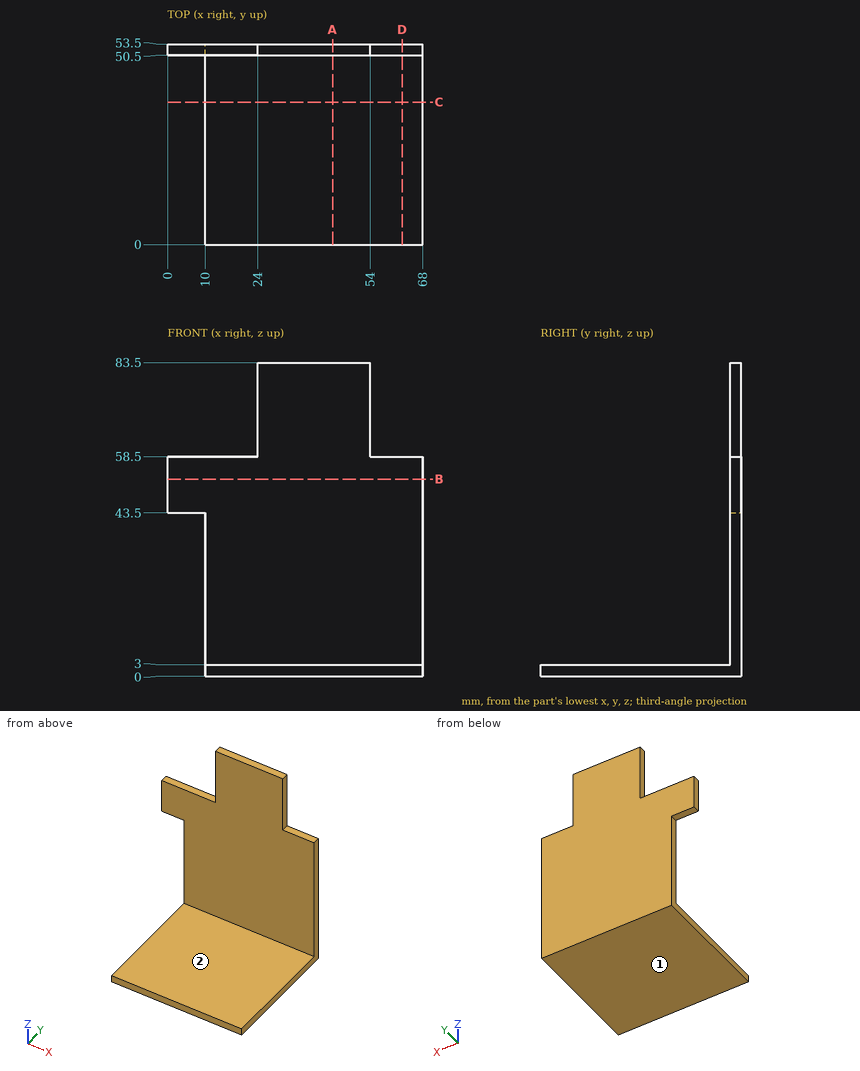
Check sheet for the drawn part. Datum: minimum x, y, z corner. Units: mm. A direction names the side the tool comes from. Give positions to 0.01 mm unless a question says otherwise; leave off trailing zeros. Write each loop counter-clockwise with the first axis right and the second up, starting at its lowest first coordinate (ties: lowest second). Pieces come first, ordered by that corner, then holes.
(1) Gauge pin test, flat ends, axial feed: pin 1 (12 mm diameter, centred on y = 21.5, z = 10, fed in from -X); pin 2 (12 mm diameter, centred on x = 40.5, z = 26, fed in from -Y); pin 3 (3 mm diameter, centred on x = 59, y = 14, fed in from +Z); pin 4 (2.5 mm diameter, centred on x = 14, y = 52.5, fed in from +Z). Record the tip position at first contact, or that the pin passes through.
(2) Cross-section at D-D (x = 62.5). Enter the section's corners in (y, z).
(3) Cross-section at C-C (y = 38). Enter the section's corners in (x, z), plus the area to 3 significant figures.
(4) Cross-section at B-B (z = 52.5). Enter the section's corners in (x, y), plus the area to 3 significant figures.
(5) Material ranges on line 1 (Y direction, x = 48, z = 69.5); line 2 (Z direction, x = 45, y = 23.5), recorded low to high.
(6) Cross-section at A-A (x = 44). Enter the section's corners in (y, z).
(7) Access from +Z, -Z, +X, -X, +Y, -Y to the whole of each face (thin tool, end or side, straight path). Record for the marked faces 1 and 2.
Worked out:
1. pin 1: passes through
1. pin 2: stops at y = 50.5
1. pin 3: stops at z = 3
1. pin 4: stops at z = 58.5
2. outline: (0, 0) - (53.5, 0) - (53.5, 58.5) - (50.5, 58.5) - (50.5, 3) - (0, 3) - close
3. outline: (10, 0) - (68, 0) - (68, 3) - (10, 3) - close
3. area: 174 mm2
4. outline: (0, 50.5) - (68, 50.5) - (68, 53.5) - (0, 53.5) - close
4. area: 204 mm2
5. line 1: y = 50.5 to 53.5
5. line 2: z = 0 to 3
6. outline: (0, 0) - (53.5, 0) - (53.5, 83.5) - (50.5, 83.5) - (50.5, 3) - (0, 3) - close
7. face 1: -Z, +X, -X, +Y, -Y
7. face 2: +Z, +X, -X, -Y
